from build123d import *

# Parameters (mm, degrees)
SKETCH1_W               = 85
SKETCH1_H               = 56
PCB_DEPTH               = 1.4
M2_5_HOLE_1_DEPTH       = 102.798624745
M2_5_HOLE_1_DEPTH_BACK  = 102.798624745
SKETCH2_R               = 1.375
M2_5_HOLE_2_DEPTH       = 102.798624745
M2_5_HOLE_2_DEPTH_BACK  = 102.798624745
SKETCH3_R               = 1.375
M2_5_HOLE_3_DEPTH       = 102.798624745
M2_5_HOLE_3_DEPTH_BACK  = 102.798624745
SKETCH4_R               = 1.375
M2_5_HOLE_4_DEPTH       = 102.798624745
M2_5_HOLE_4_DEPTH_BACK  = 102.798624745
SKETCH5_R               = 1.375
GPIO_HEADER_40PIN_START = 1.4
SKETCH6_W               = 50.8
SKETCH6_H               = 5.1
GPIO_HEADER_40PIN_DEPTH = 8.5
USB_PAIR_1_START        = 1.4
SKETCH7_W               = 17.4
SKETCH7_H               = 14.6
USB_PAIR_1_DEPTH        = 16
USB_PAIR_2_START        = 1.4
SKETCH8_W               = 17.4
SKETCH8_H               = 14.6
USB_PAIR_2_DEPTH        = 16
ETHERNET_RJ45_START     = 1.4
SKETCH9_W               = 21.4
SKETCH9_H               = 16
ETHERNET_RJ45_DEPTH     = 13.5
SOC_BCM2837B0_START     = 1.4
SKETCH10_W              = 14
SKETCH10_H              = 14
SOC_BCM2837B0_DEPTH     = 1.3
HDMI_START              = 1.4
SKETCH11_W              = 15.1
SKETCH11_H              = 11.6
HDMI_DEPTH              = 6.4
MICRO_USB_POWER_START   = 1.4
SKETCH12_W              = 8
SKETCH12_H              = 5.6
MICRO_USB_POWER_DEPTH   = 2.6
AUDIO_JACK_START        = 1.4
SKETCH13_W              = 7
SKETCH13_H              = 12.5
AUDIO_JACK_DEPTH        = 6
WIFI_SHIELD_START       = 1.4
SKETCH14_W              = 10
SKETCH14_H              = 10
WIFI_SHIELD_DEPTH       = 1.5
LAN_CHIP_START          = 1.4
SKETCH15_W              = 9
SKETCH15_H              = 9
LAN_CHIP_DEPTH          = 1
SKETCH16_W              = 13
SKETCH16_H              = 12
MICROSD_SLOT_DEPTH      = 1.5


with BuildPart() as part:
    # Sketch1 → PCB (new body)
    with BuildSketch(Plane(origin=(0, 0, 0), x_dir=(1, 0, 0), z_dir=(0, 1, 0))):
        with Locations((42.5, 28)):
            Rectangle(SKETCH1_W, SKETCH1_H)
    extrude(amount=PCB_DEPTH)

    # Sketch2 → M2_5_hole_1 (cut, two sides: drawn at the far end of the back side and taken through both)
    with BuildSketch(Plane(origin=(0, 0, 0), x_dir=(1, 0, 0), z_dir=(0, 1, 0)).offset(-M2_5_HOLE_1_DEPTH_BACK)):
        with Locations(Location((3.5, 3.5, 0), (0, 0, 270))):
            Circle(SKETCH2_R)
    extrude(amount=M2_5_HOLE_1_DEPTH + M2_5_HOLE_1_DEPTH_BACK, mode=Mode.SUBTRACT)

    # Sketch3 → M2_5_hole_2 (cut, two sides: drawn at the far end of the back side and taken through both)
    with BuildSketch(Plane(origin=(0, 0, 0), x_dir=(1, 0, 0), z_dir=(0, 1, 0)).offset(-M2_5_HOLE_2_DEPTH_BACK)):
        with Locations(Location((61.5, 3.5, 0), (0, 0, 270))):
            Circle(SKETCH3_R)
    extrude(amount=M2_5_HOLE_2_DEPTH + M2_5_HOLE_2_DEPTH_BACK, mode=Mode.SUBTRACT)

    # Sketch4 → M2_5_hole_3 (cut, two sides: drawn at the far end of the back side and taken through both)
    with BuildSketch(Plane(origin=(0, 0, 0), x_dir=(1, 0, 0), z_dir=(0, 1, 0)).offset(-M2_5_HOLE_3_DEPTH_BACK)):
        with Locations(Location((3.5, 52.5, 0), (0, 0, 270))):
            Circle(SKETCH4_R)
    extrude(amount=M2_5_HOLE_3_DEPTH + M2_5_HOLE_3_DEPTH_BACK, mode=Mode.SUBTRACT)

    # Sketch5 → M2_5_hole_4 (cut, two sides: drawn at the far end of the back side and taken through both)
    with BuildSketch(Plane(origin=(0, 0, 0), x_dir=(1, 0, 0), z_dir=(0, 1, 0)).offset(-M2_5_HOLE_4_DEPTH_BACK)):
        with Locations(Location((61.5, 52.5, 0), (0, 0, 270))):
            Circle(SKETCH5_R)
    extrude(amount=M2_5_HOLE_4_DEPTH + M2_5_HOLE_4_DEPTH_BACK, mode=Mode.SUBTRACT)

    # Sketch6 → GPIO_header_40pin (add)
    with BuildSketch(Plane(origin=(0, 0, 0), x_dir=(1, 0, 0), z_dir=(0, 1, 0)).offset(GPIO_HEADER_40PIN_START)):
        with Locations((32.5, 52.55)):
            Rectangle(SKETCH6_W, SKETCH6_H)
    extrude(amount=GPIO_HEADER_40PIN_DEPTH)

    # Sketch7 → USB_pair_1 (add)
    with BuildSketch(Plane(origin=(0, 0, 0), x_dir=(1, 0, 0), z_dir=(0, 1, 0)).offset(USB_PAIR_1_START)):
        with Locations((78.7, 29)):
            Rectangle(SKETCH7_W, SKETCH7_H)
    extrude(amount=USB_PAIR_1_DEPTH)

    # Sketch8 → USB_pair_2 (add)
    with BuildSketch(Plane(origin=(0, 0, 0), x_dir=(1, 0, 0), z_dir=(0, 1, 0)).offset(USB_PAIR_2_START)):
        with Locations((78.7, 47)):
            Rectangle(SKETCH8_W, SKETCH8_H)
    extrude(amount=USB_PAIR_2_DEPTH)

    # Sketch9 → Ethernet_RJ45 (add)
    with BuildSketch(Plane(origin=(0, 0, 0), x_dir=(1, 0, 0), z_dir=(0, 1, 0)).offset(ETHERNET_RJ45_START)):
        with Locations((76.3, 10.25)):
            Rectangle(SKETCH9_W, SKETCH9_H)
    extrude(amount=ETHERNET_RJ45_DEPTH)

    # Sketch10 → SoC_BCM2837B0 (add)
    with BuildSketch(Plane(origin=(0, 0, 0), x_dir=(1, 0, 0), z_dir=(0, 1, 0)).offset(SOC_BCM2837B0_START)):
        with Locations((28, 24.5)):
            Rectangle(SKETCH10_W, SKETCH10_H)
    extrude(amount=SOC_BCM2837B0_DEPTH)

    # Sketch11 → HDMI (add)
    with BuildSketch(Plane(origin=(0, 0, 0), x_dir=(1, 0, 0), z_dir=(0, 1, 0)).offset(HDMI_START)):
        with Locations((32.05, 4.8)):
            Rectangle(SKETCH11_W, SKETCH11_H)
    extrude(amount=HDMI_DEPTH)

    # Sketch12 → Micro_USB_power (add)
    with BuildSketch(Plane(origin=(0, 0, 0), x_dir=(1, 0, 0), z_dir=(0, 1, 0)).offset(MICRO_USB_POWER_START)):
        with Locations((10.6, 1.8)):
            Rectangle(SKETCH12_W, SKETCH12_H)
    extrude(amount=MICRO_USB_POWER_DEPTH)

    # Sketch13 → Audio_jack (add)
    with BuildSketch(Plane(origin=(0, 0, 0), x_dir=(1, 0, 0), z_dir=(0, 1, 0)).offset(AUDIO_JACK_START)):
        with Locations((53.5, 5.25)):
            Rectangle(SKETCH13_W, SKETCH13_H)
    extrude(amount=AUDIO_JACK_DEPTH)

    # Sketch14 → WiFi_shield (add)
    with BuildSketch(Plane(origin=(0, 0, 0), x_dir=(1, 0, 0), z_dir=(0, 1, 0)).offset(WIFI_SHIELD_START)):
        with Locations((11, 29)):
            Rectangle(SKETCH14_W, SKETCH14_H)
    extrude(amount=WIFI_SHIELD_DEPTH)

    # Sketch15 → LAN_chip (add)
    with BuildSketch(Plane(origin=(0, 0, 0), x_dir=(1, 0, 0), z_dir=(0, 1, 0)).offset(LAN_CHIP_START)):
        with Locations((59.5, 16.5)):
            Rectangle(SKETCH15_W, SKETCH15_H)
    extrude(amount=LAN_CHIP_DEPTH)

    # Sketch16 → MicroSD_slot (add)
    with BuildSketch(Plane(origin=(0, 0, 0), x_dir=(1, 0, 0), z_dir=(0, 1, 0))):
        with Locations((4, 28)):
            Rectangle(SKETCH16_W, SKETCH16_H)
    extrude(amount=-MICROSD_SLOT_DEPTH)


solid = part.part
Build history of the part. All positions in model axes, mm. A direction names the side the tool comes from. Coordinates: 2 decimals unless noted, no trailing zeros. Order: outer loops, then holes, each group sorted by start corner. A loop starts at its lowest first (then second) coordinate and runs counter-clockwise, first axis right, second up. Notation, with made-up numbers: (83.25, -9.5) -> (94.25, -9.5) arc R25 ccw to (94.25, 17.5) -> close; hole circle Ø11 at (35, 32). An arc over 180 degrees is marked (long way). One line per item, written item: value.
(1) Drop flat-ended pins along their axis: pin 1 Ø7.5 at (x, z) = (54.5, -7.5) entering from +Y; pin 2 Ø0.8 at (y, z) = (2, -16) entering from -X; pin 3 Ø1.6 at (x, y) = (3.5, -0.5) entering from -Z; pin 4 Ø2.5 at (x, y) = (34, 6.5) entering from -Z. Give the stop position or say it passes through.
Checked values:
pin 1: y = 7.4
pin 2: x = 55
pin 3: z = -56
pin 4: z = -55.1
(2) Slice it at B-B, the plane z = -52.5. List the corners of the cut face in (x, y) (3 decimals), plus the area to 4 significant figures.
Checked values:
outline: (0, 0) -> (2.125, 0) -> (2.125, 1.4) -> (0, 1.4) -> close; (4.875, 0) -> (60.125, 0) -> (60.125, 1.4) -> (57.9, 1.4) -> (57.9, 9.9) -> (7.1, 9.9) -> (7.1, 1.4) -> (4.875, 1.4) -> close; (62.875, 0) -> (85, 0) -> (85, 1.4) -> (87.4, 1.4) -> (87.4, 17.4) -> (70, 17.4) -> (70, 1.4) -> (62.875, 1.4) -> close
area: 821.5 mm2
(3) Slice it at A-A, the plane x = 3.5. List the corners of the cut face in (y, z) (3 decimals), plus the area to 3 significant figures.
Checked values:
outline: (-1.5, -34) -> (0, -34) -> (0, -51.125) -> (1.4, -51.125) -> (1.4, -4.875) -> (0, -4.875) -> (0, -22) -> (-1.5, -22) -> close; (0, -56) -> (1.4, -56) -> (1.4, -53.875) -> (0, -53.875) -> close; (0, -2.125) -> (1.4, -2.125) -> (1.4, 0) -> (0, 0) -> close
area: 88.7 mm2
(4) Mould opens along X. For faces 1 (the flat face through (7.1, 6, -53)), 2 (the flat face through (79, 9, -54.3)), 3 (the flat face through (24.5, 5, -5)), 4 (the flat face through (57, 4, -5)) say: pulls with the +X half, pulls with the -X half, needs draft (parallel to the pull), parting line crosses it, or undercut.
Checked values:
face 1: pulls with the -X half
face 2: needs draft
face 3: undercut
face 4: undercut
(5) Slice it at D-D, the plane z = -20. List the corners of the cut face in (x, y), plus the area to 3 significant figures.
Checked values:
outline: (0, 0) -> (85, 0) -> (85, 1.4) -> (64, 1.4) -> (64, 2.4) -> (55, 2.4) -> (55, 1.4) -> (35, 1.4) -> (35, 2.7) -> (21, 2.7) -> (21, 1.4) -> (0, 1.4) -> close
area: 146 mm2
(6) Tool access for faces 5 (the flat face through (11, 2.9, -29)), 6 (the flat face through (79, 9, -36.3)), 7 (the flat face through (59, 2.4, -17)), 8 (the flat face through (39.6, 5, -5)), 9 (the flat face through (70, 9, -47)): list every direction of +Z, -Z, +X, -X, +Y, -Y with a clear straight run to the whole face (end or side of a thin tool).
Checked values:
face 5: -X, +Y
face 6: +X, -X, +Y
face 7: +Y
face 8: +Z, +Y
face 9: -Z, +Y
(7) Slice it at C-C, the plane y = 9. List the corners of the cut face in (x, z).
Checked values:
outline: (7.1, -55.1) -> (57.9, -55.1) -> (57.9, -50) -> (7.1, -50) -> close; (65.6, -18.25) -> (87, -18.25) -> (87, -2.25) -> (65.6, -2.25) -> close; (70, -54.3) -> (87.4, -54.3) -> (87.4, -39.7) -> (70, -39.7) -> close; (70, -36.3) -> (87.4, -36.3) -> (87.4, -21.7) -> (70, -21.7) -> close
(8) Probe line 1 (Z direction, x = 3.5, y = 0.45) (3 decimals); line 2 (X direction, y = 0.4, z = -52.5) (3 decimals); line 3 (Z direction, x = 74, y = 10). List the from-to ranges inside material, lowest first. Write a range as [from, to].
Checked values:
line 1: [-56, -53.875], [-51.125, -4.875], [-2.125, 0]
line 2: [0, 2.125], [4.875, 60.125], [62.875, 85]
line 3: [-54.3, -39.7], [-36.3, -21.7], [-18.25, -2.25]
